Here's how the part is built. I have some questions about the finished solid (model axes, mm). Give positions to 0.01 mm unless a question says otherwise; leave off trailing zeros. Loops run counter-clockwise (first coordinate to the right, second up) from the corner with the lowest first, then second, coordinate; pieces in that order, holes last.
Q1. Suppose I cut it at A-A (z = 2.7). Count the separate pieces of the cut face and the enclosed holes in it, and give its area (3 significant figures).
Q2. Suppose I cut it at B-B (x = -51.5). List the corners of the cut face in (y, z) for me.
Q3. I need wall thicknesses on probe 1 along Y at (x, z) = (-10.5, 3.65); probe 2 along X at (y, z) = (-84.5, 3.4); probe 3 along X at (y, z) = (18, 2.85). Which ranges of each line are inside material? Lowest first, please.
```python
from build123d import *

# Parameters (mm, degrees)
SKETCH_1_W          = 110
SKETCH_1_H          = 126
EXTRUDE_1_DEPTH     = 4
SKETCH_2_R          = 2.7
SKETCH_2_R_2        = 3.25
SKETCH_2_R_3        = 4
SKETCH_2_R_4        = 2.1
CUT_EXTRUDE_2_DEPTH = 4
CUT_EXTRUDE_3_DEPTH = 4


with BuildPart() as part:
    # 草图1 → 凸台-拉伸1 (new body)
    with BuildSketch(Plane.XY):
        with Locations((-12.266115935, -37.027805236)):
            Rectangle(SKETCH_1_W, SKETCH_1_H)
    extrude(amount=EXTRUDE_1_DEPTH)

    # 草图2 → 切除-拉伸2 (cut)
    with BuildSketch(Plane.XY.offset(4)):
        with Locations((12.733884065, -48.027805236)):
            Circle(SKETCH_2_R)
        with Locations((32.733884065, -82.727805236)):
            Circle(SKETCH_2_R)
        with Locations((-37.266115935, -48.027805236)):
            Circle(SKETCH_2_R)
        with Locations((-57.266115935, -82.727805236)):
            Circle(SKETCH_2_R)
        with Locations((-12.266115935, -80.027805236)):
            Circle(SKETCH_2_R_2)
        with Locations((-12.266115935, -4.027805236)):
            Circle(SKETCH_2_R_3)
        with Locations((-12.266115935, 10.972194764)):
            Circle(SKETCH_2_R_4)
        with Locations((-12.266115935, -19.027805236)):
            Circle(SKETCH_2_R_4)
    extrude(amount=-CUT_EXTRUDE_2_DEPTH, mode=Mode.SUBTRACT)

    # 草图3 → 切除-拉伸3 (cut)
    with BuildSketch(Plane.XY.offset(4)):
        Polygon((-67.266115935, 5.972194764), (-47.266115935, 25.972194764), (-67.266115935, 25.972194764), align=None)
        Polygon((22.733884065, 25.972194764), (42.733884065, 5.972194764), (42.733884065, 25.972194764), align=None)
    extrude(amount=-CUT_EXTRUDE_3_DEPTH, mode=Mode.SUBTRACT)


solid = part.part
```
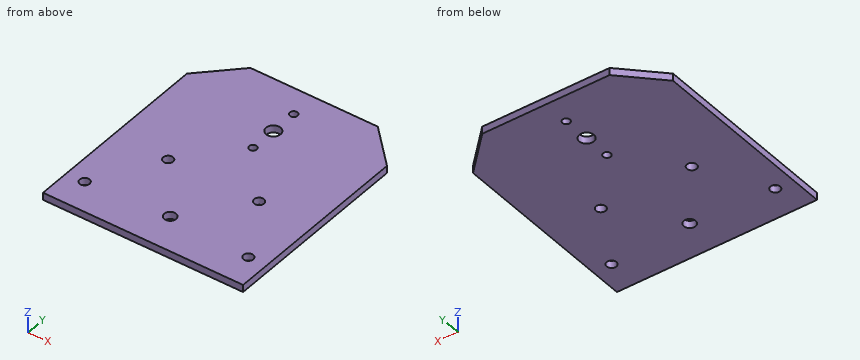
Solutions:
1. separate pieces: 1
1. enclosed holes: 8
1. area: 13,300 mm2
2. outline: (-100.03, 0) - (21.74, 0) - (21.74, 4) - (-100.03, 4) - close
3. probe 1: y = -100.03 to -82.76, -77.3 to -20.16, -17.89 to -7.62, -0.44 to 9.84, 12.11 to 25.97
3. probe 2: x = -67.27 to -59.3, -55.23 to 30.7, 34.77 to 42.73
3. probe 3: x = -55.24 to 30.71
